Check sheet for the drawn part. Datum: minimum x, y, z corner. Units: mm. Round coordinates to 2 decimals unless told otherwise and drop trailing zeros. Order: outer loops, then holes, each group sorted by start corner. A loop starts at its lowest first (then second) coordinate and runs counter-clockwise, first axis right, second up. Notation, with made-up numbers: (-22.75, 17) -> (-4.75, 17) arc R13 cw to (-4.75, 24) -> close; hole circle Ø6 at (-32, 57). An arc over 180 degrees is marked (long way). Answer in a Markdown table with one row per item.
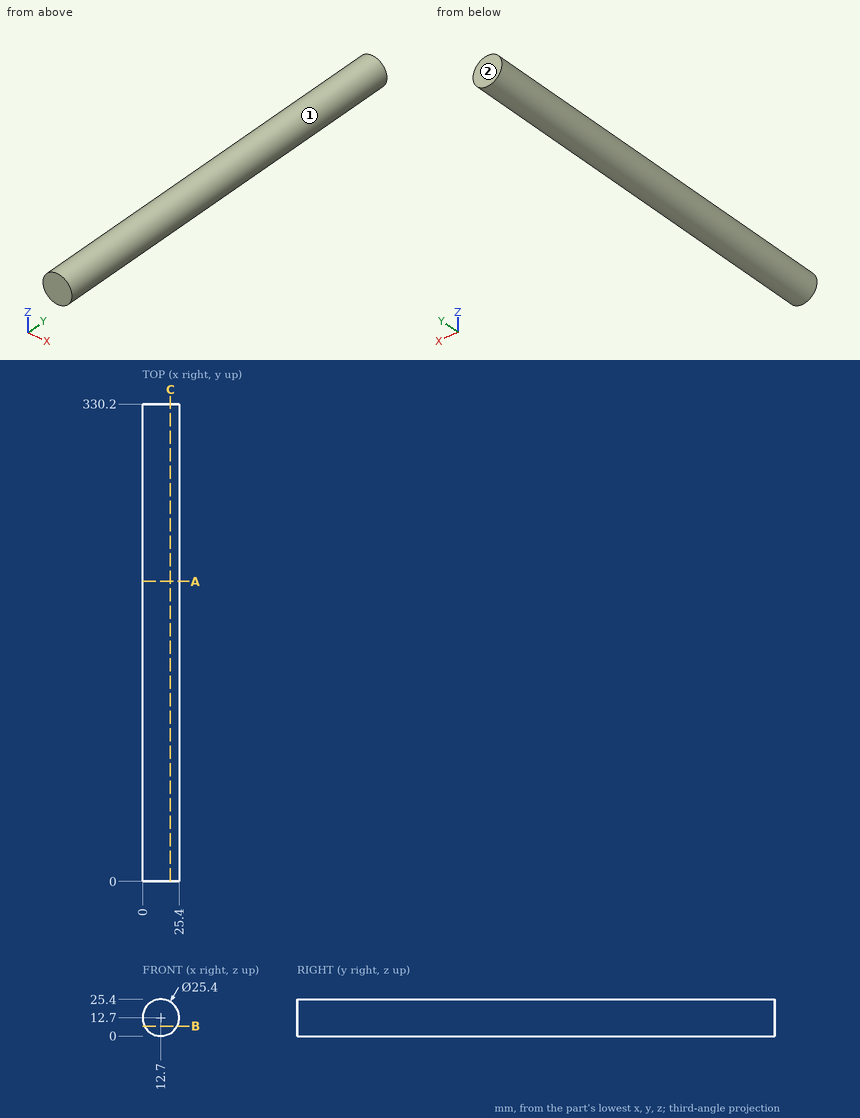
(1) Draft check along X on the marked faces 1 and 2. Enter one of: pulls with the +X half, pulls with the -X half, needs draft (parallel to the pull), parting line crosses it, or undercut.
Solutions:
| item | result |
|---|---|
| face 1 | parting line crosses it |
| face 2 | needs draft |
(2) Depth check by flat-ended pin: pin 1 Ø6 at (y, z) = (212, 6.5) entering from +X; pin 2 Ø6 at (y, z) = (41, 17) entering from -X; pin 3 Ø1 at (x, y) = (6.5, 76.5) entering from +Z. Enter the tip coordinate at first touch or a pass-through.
Solutions:
| item | result |
|---|---|
| pin 1 | x = 24.99 |
| pin 2 | x = 0.07 |
| pin 3 | z = 24.05 |
(3) Section check C-C on x = 19.25. Record the boundary of the cut face in (y, z).
Solutions:
| item | result |
|---|---|
| outline | (0, 1.82) -> (330.2, 1.82) -> (330.2, 23.58) -> (0, 23.58) -> close |
(4) Section check A-A on y = 207.5. Record the boundary of the cut face in (x, z), plus the area to 3 significant figures.
Solutions:
| item | result |
|---|---|
| outline | circle Ø25.4 at (12.7, 12.7) |
| area | 507 mm^2 |
(5) Scan lines: probe 1 along Z at (x, y) = (13.5, 265); probe 2 along X at (y, z) = (242, 19); probe 3 along Z at (x, y) = (22.25, 229). Record each from-to range of solid material in increasing order. Write a range as from..to.
Solutions:
| item | result |
|---|---|
| probe 1 | 0.03..25.37 |
| probe 2 | 1.67..23.73 |
| probe 3 | 4.33..21.07 |
(6) Section check B-B on z = 6.75. Record the boundary of the cut face in (x, y).
Solutions:
| item | result |
|---|---|
| outline | (1.48, 0) -> (23.92, 0) -> (23.92, 330.2) -> (1.48, 330.2) -> close |
